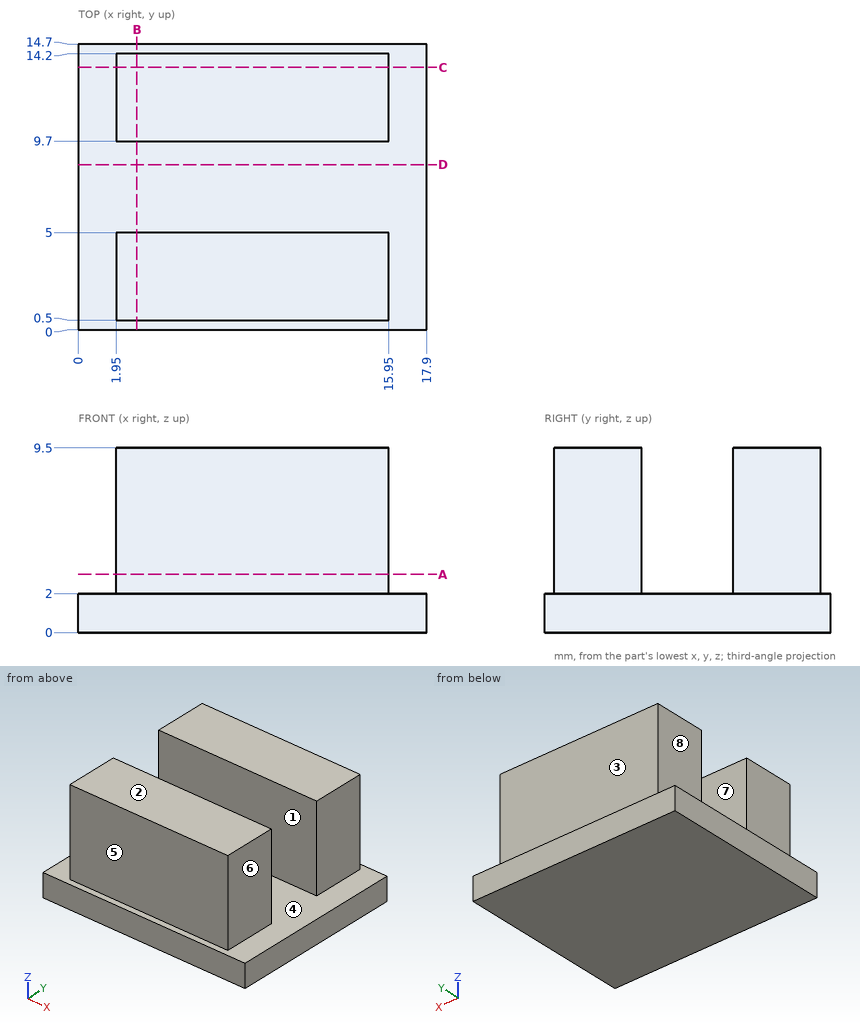
For this review, use the dimensioned drawing (mm, ordinates from the lowest corner) and the shaded views. A direction names the side the tool comes from. Give positions to 0.01 mm unless a question says otherwise; leave off trailing zeros. Order: outer loops, then holes, each group sorted by start corner. A loop starts at its lowest first (then second) coordinate and runs counter-clockwise, first axis right, second up. Notation, with made-up numbers: (72.25, 36.5) - (80.25, 36.5) arc R21 cw to (80.25, 64.5) - close; hole circle Ø10 at (10.25, 28). An arc over 180 degrees is marked (long way). Use a Markdown table: item, result. Add a question column.
(1) Add section B-B on x = 3. Give the boundary of the cut face in (y, z), then the cut area to 3 significant figures.
(2) Wall thickness on probe 1 along Y at (x, z) = (3.5, 8.5); probe 2 along X at (y, z) = (3, 4.5); probe 3 along Z at (x, y) = (3.5, 7.25): over which ranges is each line inside the solid? List them lowest first. Write a range as [from, to].
(3) Machinability: for the marked faces 5, 6, 7 and 8, which of the approach directions +Z, -Z, +X, -X, +Y, -Y give a long, thin tool a straight path to every point of the face, cutting with its end or side? Answer none if there is none.
(4) Clearance check with flat-ended pins moving along their axes: P1, Ø2, axis at x = 3, y = 6.5, coming from the +Z side; P2, Ø3, axis at y = 3.5, z = 5.5, coming from the +X side; P3, Ø3, axis at y = 4.5, z = 5.5, coming from the -X side; P4, Ø7.5, axis at x = 8, y = 9, coming from the +Z side. State where each tip first meets the part, or that it passes through.
(5) Mouldability with a two-part tool opening along Y and no side actions: class the marked faces 1, 2, 3 and 4 as +Y half, -Y half, draft (parallel to the pull), parting line (faces both ways), or undercut.
(6) Add section A-A on z = 3. Give the boundary of the cut face in (x, y), then the cut area to 3 significant figures.
(7) Add section D-D on y = 8.5. Give the boundary of the cut face in (x, z).
(8) Add section C-C on y = 13.5. Give the boundary of the cut face in (x, z), then the cut area to 3 significant figures.
Report:
| question | item | result |
|---|---|---|
| 1 | outline | (0, 0) - (14.7, 0) - (14.7, 2) - (14.2, 2) - (14.2, 9.5) - (9.7, 9.5) - (9.7, 2) - (5, 2) - (5, 9.5) - (0.5, 9.5) - (0.5, 2) - (0, 2) - close |
| 1 | area | 96.9 mm² |
| 2 | probe 1 | y = [0.5, 5], [9.7, 14.2] |
| 2 | probe 2 | x = [1.95, 15.95] |
| 2 | probe 3 | z = [0, 2] |
| 3 | face 5 | +Z, +X, -X, -Y |
| 3 | face 6 | +Z, +X, +Y, -Y |
| 3 | face 7 | +Z, +X, -X |
| 3 | face 8 | +Z, -X, +Y, -Y |
| 4 | P1 | stops at z = 2 |
| 4 | P2 | stops at x = 15.95 |
| 4 | P3 | stops at x = 1.95 |
| 4 | P4 | stops at z = 9.5 |
| 5 | face 1 | undercut |
| 5 | face 2 | draft |
| 5 | face 3 | +Y half |
| 5 | face 4 | undercut |
| 6 | outline | (1.95, 0.5) - (15.95, 0.5) - (15.95, 5) - (1.95, 5) - close; (1.95, 9.7) - (15.95, 9.7) - (15.95, 14.2) - (1.95, 14.2) - close |
| 6 | area | 126 mm² |
| 7 | outline | (0, 0) - (17.9, 0) - (17.9, 2) - (0, 2) - close |
| 8 | outline | (0, 0) - (17.9, 0) - (17.9, 2) - (15.95, 2) - (15.95, 9.5) - (1.95, 9.5) - (1.95, 2) - (0, 2) - close |
| 8 | area | 141 mm² |
